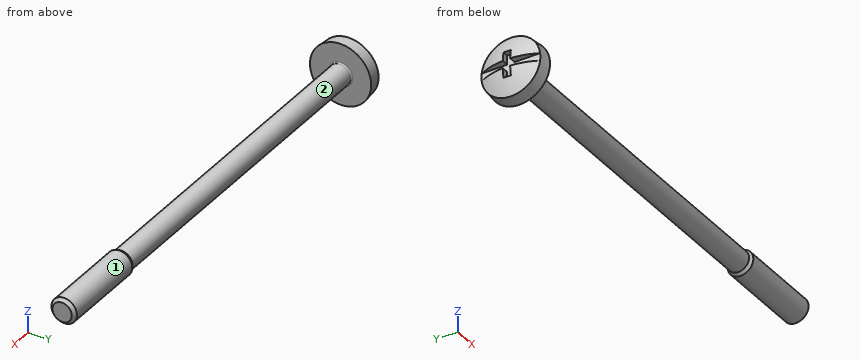
```python
from build123d import *

# Parameters (mm, degrees)
CUT_EXTRUDE1_DEPTH = 0.6


with BuildPart() as part:
    # Sketch1 → Revolve1 (revolve)
    with BuildSketch(Plane.XY):
        with BuildLine():
            Line((-1.04, 2.30901179), (0, 2.4))
            Line((0, 2.4), (0, 0.945))
            ThreePointArc((0, 0.945), (0.029289322, 0.874289322), (0.1, 0.845))
            Line((0.1, 0.845), (26.731532125, 0.845))
            Line((26.731532125, 0.845), (27, 1))
            Line((27, 1), (33.7545, 1))
            Line((33.7545, 1), (34, 0.7545))
            Line((34, 0.7545), (34, 0))
            Line((34, 0), (-1.6, 0))
            ThreePointArc((-1.6, 0), (-1.457999714, 1.187974689), (-1.04, 2.30901179))
        make_face()
    revolve(axis=Axis((34, 0, 0), (-1, 0, 0)))

    # Sketch2 → Cut-Extrude1 (cut)
    with BuildSketch(Plane(origin=(-1.04, 0, 0), x_dir=(0, 0, -1), z_dir=(1, 0, 0))):
        Polygon((-1, 0.29), (-1, -0.29), (-0.29, -0.29), (-0.29, -2.5), (0.29, -2.5), (0.29, -0.29), (1, -0.29), (1, 0.29), (0.29, 0.29), (0.29, 2.5), (-0.29, 2.5), (-0.29, 0.29), align=None)
    extrude(amount=-CUT_EXTRUDE1_DEPTH, mode=Mode.SUBTRACT)


solid = part.part
```
The listing builds one solid part. Answer for the finished solid, in the listing's coordinates (mm). Face numbers are marked on the shaded views. Round coordinates to 2 decimals unless told otherwise and drop trailing zeros. Loops run counter-clockwise (first coordinate to the right, second up) from the corner with the lowest first, then second, coordinate; pieces in that order, holes last. Notation, with made-up numbers: (44, 13) - (70, 13) arc R17 ccw to (70, 46) - close; hole circle Ø9 at (56.5, 44.25). An arc over 180 degrees is marked (long way). Use one line per item in the form item = value. Start each with the question number.
1. Given pin 1 Ø1 at (y, z) = (-0.5, -1) entering from -X; pin 2 Ø0.6 at (x, z) = (-1.5, -0.5) entering from -Y; pin 3 Ø1 at (x, z) = (12.5, 0) entering from +Y (3 decimals), each flat-ended and moving along its own axis, determine where each tip first touches the part or whether it passes through.
2. For a pull along X with two mould halves and no side action, classify the marked faces 1 and 2 as pulls with the +X half, pulls with the -X half, needs draft (parallel to the pull), parting line crosses it, or undercut.
3. The part is cut by section C-C on x = 2. Determine the outline of the cut face in (y, z) (3 decimals).
4. Consider line 1 (X direction, y = -0.6, z = 0.15); line 2 (Y direction, x = 22, z = 0.1); line 3 (Z direction, x = 12, y = 0.75). Determine where each line is inside the solid, lowest interval first. Write a range as [from, to].
Geometry check:
q1.pin_1 = -1.56
q1.pin_2 = -1.91
q1.pin_3 = 0.845
q2.face_1 = needs draft
q2.face_2 = undercut
q3.outline = circle Ø1.69 at (0, 0)
q4.line_1 = [-1.04, 34]
q4.line_2 = [-0.84, 0.84]
q4.line_3 = [-0.39, 0.39]
